Study the drawing (mm; zero at the part's minimum x, y, z) and answer. A direction names the side the tool comes from. Round coordinates to 2 decimals unless told otherwise and drop trailing zeros. Loops run counter-clockwise (first coordinate to the right, second up) from the corner with the lowest first, then second, coordinate; pieces in that order, holes last. Notation, with made-up numbers: (-9.75, 59) -> (35.25, 59) arc R15 cw to (35.25, 80) -> close; hole circle Ø11 at (-27, 12.5). An arc over 180 degrees is marked (long way). Write each question's results on one line, items separated by ' | '. Start each with the question number.
(1) The part is cut by section B-B (x = 20). Determine the outline of the cut face in (y, z), plus the area to 3 significant figures.
(2) Flat-ended cylindrical pins translate along their axes: pin 1 (2.5 mm diameter, centred on x = 20, z = 4, fed in from +Y); pin 2 (2 mm diameter, centred on y = 5, z = 16, fed in from -X); pin 3 (2 mm diameter, centred on y = 1, z = 17.5, fed in from -X); pin 4 (4 mm diameter, centred on y = 3, z = 31, fed in from +X). Find the tip coordinate at first contact, or state that the pin passes through.
(3) For the marked faces 4 and 5, determine the directions among +Z, -Z, +X, -X, +Y, -Y from which every point of the face is accessible in a straight line to the end or side of a thin tool.
(4) The part is cut by section C-C (z = 20). Determine the outline of the cut face in (x, y).
(5) The part is cut by section D-D (x = 4). Determine the outline of the cut face in (y, z).
(6) Determine the mould class of the marked faces 1, 2 and 3 for opening direction X: released by +X, released by -X, zero draft, split by the parting line, or undercut.
(7) The part is cut by section A-A (z = 36). Determine the outline of the cut face in (x, y).
(8) Straight lines are drawn through the part: probe 1 along X at (y, z) = (3, 20); probe 2 along X at (y, z) = (4.25, 36); probe 3 along Y at (x, z) = (24, 30). For each, find the intervals that lie inside material, in ascending order.
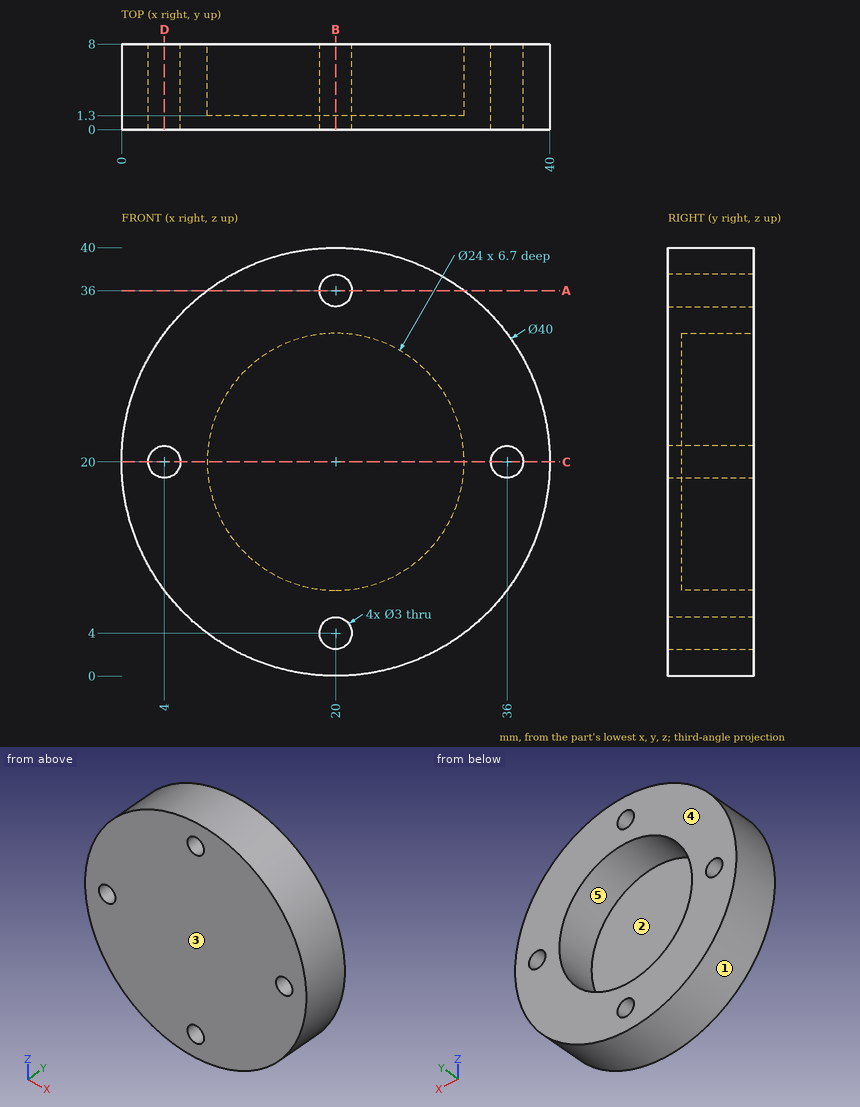
Checked values:
1) outline: (0, 0) -> (8, 0) -> (8, 2.5) -> (0, 2.5) -> close; (0, 5.5) -> (8, 5.5) -> (8, 8) -> (1.3, 8) -> (1.3, 32) -> (8, 32) -> (8, 34.5) -> (0, 34.5) -> close; (0, 37.5) -> (8, 37.5) -> (8, 40) -> (0, 40) -> close | area: 111 mm2
2) pin 1: passes through | pin 2: stops at x = 0.23 | pin 3: stops at x = 0.06 | pin 4: stops at x = 37.86
3) face 4: +Z, -Z, +X, -X, +Y | face 5: +Y
4) outline: (0, 0) -> (2.5, 0) -> (2.5, 8) -> (0, 8) -> close; (5.5, 0) -> (34.5, 0) -> (34.5, 8) -> (32, 8) -> (32, 1.3) -> (8, 1.3) -> (8, 8) -> (5.5, 8) -> close; (37.5, 0) -> (40, 0) -> (40, 8) -> (37.5, 8) -> close
5) outline: (0, 8) -> (8, 8) -> (8, 18.5) -> (0, 18.5) -> close; (0, 21.5) -> (8, 21.5) -> (8, 32) -> (0, 32) -> close
6) face 1: split by the parting line | face 2: undercut | face 3: zero draft
7) outline: (8, 0) -> (18.5, 0) -> (18.5, 8) -> (8, 8) -> close; (21.5, 0) -> (32, 0) -> (32, 8) -> (21.5, 8) -> close
8) probe 1: x = 0 to 2.5, 5.5 to 8, 32 to 34.5, 37.5 to 40 | probe 2: x = 8 to 18.5, 21.5 to 32 | probe 3: y = 0 to 1.3
